Build history of the part. All positions in model axes, mm. Give positions to 0.01 mm unless a question says otherwise; leave off trailing zeros. Loops run counter-clockwise (first coordinate to the right, second up) from the corner with the lowest first, then second, coordinate; pieces in that order, holes last.
1) Flat gauge pin, fed straight in: P1, Ø3, axis at y = 99.52, z = 6.35, coming from the -X side. Where does the tip first touch, or does it go through?
2) Band-saw the part on A-A on z = 6.35. List the corners of the cut face in (x, y), then the cut area to 3 significant figures.
3) Two-plate mould, pull along Y, no slides. Class faces 1 (the flat face through (-23, 25, 0)), 2 (the cylindrical face through (-22.54, 21.35, 5.91)), 3 (the flat face through (-23, -78.28, 6)): +Y half, -Y half, draft (parallel to the pull), parting line (faces both ways), or undercut.
4) Wall check: line 1 (Y direction, x = -15.5, z = 6.25); line 2 (Y direction, x = -12, z = 4.75). Give the ranges that are in metal, low to high.
```python
from build123d import *

# Parameters (mm, degrees)
SKETCH1_W              = 44.45
SKETCH1_H              = 203.2
BOSS_EXTRUDE1_DEPTH    = 12.7
F_10_32_TAPPED_HOLE1_D = 4.0386


with BuildPart() as part:
    # Sketch1 → Boss-Extrude1 (new body)
    with BuildSketch(Plane.XY):
        with Locations((-22.225, 23.319966314)):
            Rectangle(SKETCH1_W, SKETCH1_H)
    extrude(amount=BOSS_EXTRUDE1_DEPTH)

    # #10-32 Tapped Hole1 (through all)
    with Locations(Plane(origin=(0, 0, 0), x_dir=(0, 0, -1), z_dir=(1, 0, 0))):
        with Locations((-6.35, 99.519966314), (-6.35, 23.319966314), (-6.35, -52.880033686)):
            Hole(F_10_32_TAPPED_HOLE1_D / 2)


solid = part.part
```
Findings below:
1. P1: passes through
2. outline: (-44.45, -78.28) - (0, -78.28) - (0, -54.9) - (-44.45, -54.9) - close; (-44.45, -50.86) - (0, -50.86) - (0, 21.3) - (-44.45, 21.3) - close; (-44.45, 25.34) - (0, 25.34) - (0, 97.5) - (-44.45, 97.5) - close; (-44.45, 101.54) - (0, 101.54) - (0, 124.92) - (-44.45, 124.92) - close
2. area: 8,490 mm2
3. face 1: draft
3. face 2: undercut
3. face 3: -Y half
4. line 1: y = -78.28 to -54.9, -50.86 to 21.3, 25.34 to 97.5, 101.54 to 124.92
4. line 2: y = -78.28 to -54.11, -51.65 to 22.09, 24.55 to 98.29, 100.75 to 124.92
